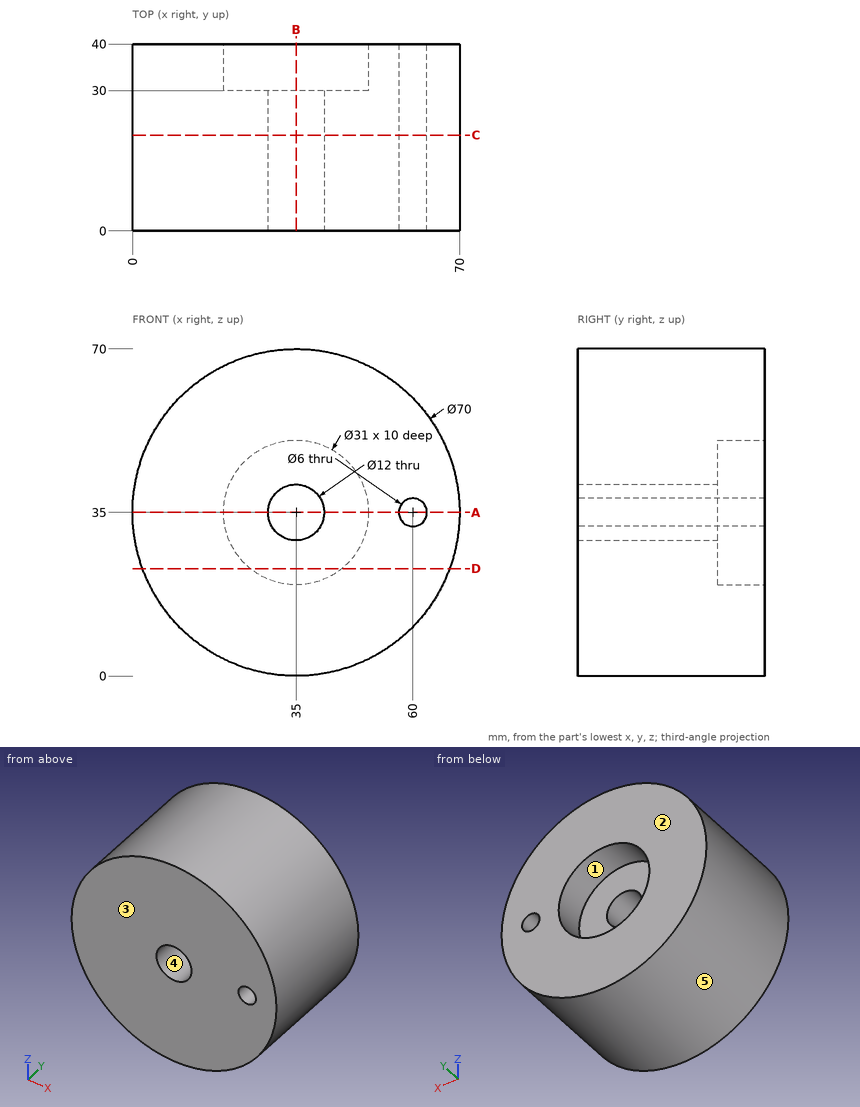
For this review, use the dimensioned drawing (mm, ordinates from the lowest corner) and the shaded views. A direction names the side the tool comes from. Give positions to 0.01 mm unless a question says otherwise; leave off trailing zeros. Order: outer loops, then holes, each group sorted by start corner. A loop starts at its lowest first (then second) coordinate and runs counter-clockwise, first axis right, second up. Notation, with made-up numbers: (-12, -21.5) -> (23, -21.5) arc R16 cw to (23, 8.5) -> close; hole circle Ø9 at (-17, 17.25). An arc over 180 degrees is marked (long way). Write item = value, one per line. Start each with the question number.
(1) Take a section at C-C (y = 20.5). Write out the cut boundary in (x, z), plus the area to 3 significant figures.
(2) Take a section at B-B (x = 35). Write out the cut boundary in (y, z), plus the area to 3 significant figures.
(3) Tool access review of the marked faces 1 and 2: name each direction out of +Z, -Z, +X, -X, +Y, -Y from which nothing blocks a thin tool from reaching the whole face with its end or side.
(4) Take a section at D-D (z = 23). Write out the cut boundary in (x, y), plus the area to 3 significant figures.
(5) For L1, parallel to X at y = 18, z = 35.5; L2, parallel to Y at x = 30, z = 41.5; L3, parallel to Z at x = 60, y = 29.5, list the stretches that pass through material, from the lowest coordinate up. Write a range as from..to.
(6) Take a section at A-A (z = 35). Write out the cut boundary in (x, y), plus the area to 3 significant figures.
(7) Draft analysis for pull direction Z (two halves, no side actions). For the marked faces 3, 4 and 5, state which applies: +Z half, -Z half, draft (parallel to the pull), parting line (faces both ways), or undercut.
(8) For pin 1 Ø2 at (y, z) = (14, 24) entering from +X; pin 2 Ø4 at (x, y) = (8, 15) entering from +Z; pin 3 Ø2 at (x, y) = (13, 21.5) entering from -Z; pin 4 Ø7 at (x, z) = (35, 35) entering from +Y, all flat-tipped, find the tip position at first contact; note any pin that passes through.
Returned:
q1.outline = circle Ø70 at (35, 35); hole circle Ø12 at (35, 35); hole circle Ø6 at (60, 35)
q1.area = 3,710 mm²
q2.outline = (0, 0) -> (40, 0) -> (40, 19.5) -> (30, 19.5) -> (30, 29) -> (0, 29) -> close; (0, 41) -> (30, 41) -> (30, 50.5) -> (40, 50.5) -> (40, 70) -> (0, 70) -> close
q2.area = 2,130 mm²
q3.face_1 = +Y
q3.face_2 = +Z, -Z, +X, -X, +Y
q4.outline = (2.12, 0) -> (67.88, 0) -> (67.88, 40) -> (44.81, 40) -> (44.81, 30) -> (25.19, 30) -> (25.19, 40) -> (2.12, 40) -> close
q4.area = 2,430 mm²
q5.L1 = 0..29.02, 40.98..57.04, 62.96..70
q5.L2 = 0..30
q5.L3 = 10.51..32, 38..59.49
q6.outline = (0, 0) -> (29, 0) -> (29, 30) -> (19.5, 30) -> (19.5, 40) -> (0, 40) -> close; (41, 0) -> (57, 0) -> (57, 40) -> (50.5, 40) -> (50.5, 30) -> (41, 30) -> close; (63, 0) -> (70, 0) -> (70, 40) -> (63, 40) -> close
q6.area = 1,890 mm²
q7.face_3 = draft
q7.face_4 = undercut
q7.face_5 = parting line
q8.pin_1 = 68.54
q8.pin_2 = 59.49
q8.pin_3 = 7
q8.pin_4 = through
